Could you check a few things on this model? Use its own coordinates, in mm. Face numbers are marked on the shaded views. Give positions to 0.01 mm unless a question says otherwise; leave off trailing zeros. Order: outer loops, then holes, each group sorted by start corner. A loop starts at its lowest first (then second) coordinate and runs counter-clockwise, first axis right, second up. Notation, with made-up numbers: (33, -10.75) -> (50, -10.75) arc R29 ccw to (50, 17.25) -> close; hole circle Ø4 at (55.25, -13). An arc over 180 degrees is marked (long way). Answer as CSV lines item,"result". Start each with the question number.
(1) Will these pins go through, and if not, where does the flat tip stop? pin 1 Ø1.5 at (x, y) = (18.5, -11) entering from -Z; pin 2 Ø6 at (x, z) = (25.5, 29) entering from +Y; pin 3 Ø6 at (y, z) = (-12, 1.5) entering from +X; pin 4 Ø2.5 at (y, z) = (1.5, 22) entering from -X.
(2) I want a section at A-A (x = 0). Please give me the cut outline in (y, z), plus the area to 3 significant figures.
(3) I want a section at B-B (y = -7). Please give me the cut outline in (x, z).
(4) I need wall thicknesses on L1, parallel to Z at x = 0, y = -10; L2, parallel to Y at x = 14.5, z = -1; L3, parallel to X at y = -4.25, z = 0.5. Which ranges of each line are inside material? Lowest first, please.
(5) We'd pull the mould along X, two halves only. Please class the marked faces 1 and 2: released by +X, released by -X, zero draft, split by the parting line, or undercut.
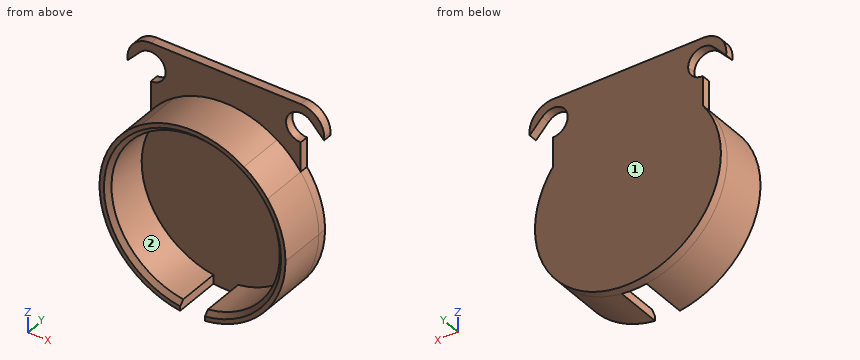
```python
from build123d import *

# Parameters (mm, degrees)
F6_R     = 28.65
F1_DEPTH = 3
F2_DEPTH = 16
F4_DEPTH = 16
F5_SIZE  = 1.5


with BuildPart() as f1:
    # F6 (on Front) → F1 (new body)
    with BuildSketch(Plane.XZ):
        with BuildLine():
            ThreePointArc((-25.5, 18.7475998464), (-9.8652800264, -30.0732231395), (31.65, 0))
            ThreePointArc((31.65, 0), (30.0732231395, 9.8652800264), (25.5, 18.7475998464))
            ThreePointArc((25.5, 18.7475998464), (21.8353418806, 22.9115766581), (17.5, 26.3718126036))
            ThreePointArc((17.5, 26.3718126036), (0, 31.65), (-17.5, 26.3718126036))
            ThreePointArc((-17.5, 26.3718126036), (-21.8353418806, 22.9115766581), (-25.5, 18.7475998464))
        make_face()
        Circle(F6_R, mode=Mode.SUBTRACT)
        Circle(F6_R)
        with BuildLine():
            ThreePointArc((-17.5, 26.3718126036), (0, 31.65), (17.5, 26.3718126036))
            Line((17.5, 26.3718126036), (17.5, 33.7475998464))
            ThreePointArc((17.5, 33.7475998464), (19.8431457505, 39.4044540959), (25.5, 41.7475998464))
            Line((25.5, 41.7475998464), (-25.5, 41.7475998464))
            ThreePointArc((-25.5, 41.7475998464), (-19.8431457505, 39.4044540959), (-17.5, 33.7475998464))
            Line((-17.5, 33.7475998464), (-17.5, 26.3718126036))
        make_face()
        with BuildLine():
            Line((-25.5, 28.7475998464), (-25.5, 25.7475998464))
            ThreePointArc((-25.5, 25.7475998464), (-19.8431457505, 28.0907455969), (-17.5, 33.7475998464))
            ThreePointArc((-17.5, 33.7475998464), (-19.8431457505, 39.4044540959), (-25.5, 41.7475998464))
            ThreePointArc((-25.5, 41.7475998464), (-31.5363482338, 38.9975998464), (-33.4227070569, 32.6382248464))
            Line((-33.4227070569, 32.6382248464), (-29.1360609327, 37.1796634958))
            ThreePointArc((-29.1360609327, 37.1796634958), (-23.6534227154, 38.3941203006), (-20.5, 33.7475998464))
            ThreePointArc((-20.5, 33.7475998464), (-21.9644660941, 30.2120659404), (-25.5, 28.7475998464))
        make_face()
        with BuildLine():
            ThreePointArc((17.5, 33.7475998464), (19.8431457505, 28.0907455969), (25.5, 25.7475998464))
            Line((25.5, 25.7475998464), (25.5, 28.7475998464))
            ThreePointArc((25.5, 28.7475998464), (20.9086865579, 35.7274586485), (29.1360609327, 37.1796634958))
            Line((29.1360609327, 37.1796634958), (33.4227070569, 32.6382248464))
            ThreePointArc((33.4227070569, 32.6382248464), (33.480653371, 33.1915676779), (33.5, 33.7475998464))
            ThreePointArc((33.5, 33.7475998464), (31.1568542495, 39.4044540959), (25.5, 41.7475998464))
            ThreePointArc((25.5, 41.7475998464), (19.8431457505, 39.4044540959), (17.5, 33.7475998464))
        make_face()
        with BuildLine():
            Line((-25.5, 25.7475998464), (-25.5, 18.7475998464))
            ThreePointArc((-25.5, 18.7475998464), (-21.8353418806, 22.9115766581), (-17.5, 26.3718126036))
            Line((-17.5, 26.3718126036), (-17.5, 33.7475998464))
            ThreePointArc((-17.5, 33.7475998464), (-19.8431457505, 28.0907455969), (-25.5, 25.7475998464))
        make_face()
        with BuildLine():
            ThreePointArc((17.5, 26.3718126036), (21.8353418806, 22.9115766581), (25.5, 18.7475998464))
            Line((25.5, 18.7475998464), (25.5, 25.7475998464))
            ThreePointArc((25.5, 25.7475998464), (19.8431457505, 28.0907455969), (17.5, 33.7475998464))
            Line((17.5, 33.7475998464), (17.5, 26.3718126036))
        make_face()
    extrude(amount=-F1_DEPTH)

    # F6 (on Front) → F2 (join)
    with BuildSketch(Plane.XZ):
        with BuildLine():
            ThreePointArc((-25.5, 18.7475998464), (-9.8652800264, -30.0732231395), (31.65, 0))
            ThreePointArc((31.65, 0), (30.0732231395, 9.8652800264), (25.5, 18.7475998464))
            ThreePointArc((25.5, 18.7475998464), (21.8353418806, 22.9115766581), (17.5, 26.3718126036))
            ThreePointArc((17.5, 26.3718126036), (0, 31.65), (-17.5, 26.3718126036))
            ThreePointArc((-17.5, 26.3718126036), (-21.8353418806, 22.9115766581), (-25.5, 18.7475998464))
        make_face()
        Circle(F6_R, mode=Mode.SUBTRACT)
    extrude(amount=F2_DEPTH)

    # F3 (on face) → F4 (cut, through all)
    with BuildSketch(Plane.XZ.offset(16)):
        with BuildLine():
            ThreePointArc((4.2, -28.3404745902), (0, -28.65), (-4.2, -28.3404745902))
            Line((-4.2, -28.3404745902), (-4.2, -31.3700892571))
            ThreePointArc((-4.2, -31.3700892571), (0, -31.65), (4.2, -31.3700892571))
            Line((4.2, -31.3700892571), (4.2, -28.3404745902))
        make_face()
    extrude(amount=-F4_DEPTH, mode=Mode.SUBTRACT)

    # F5
    f5_edges = [f1.edges().sort_by_distance(p)[0] for p in [
        (-18.714867, -16, 21.69277),
    ]]
    chamfer(f5_edges, length=F5_SIZE)


solid = f1.part
```
Final values:
1,pin 1,"z = -26.2"
1,pin 2,"y = 3"
1,pin 3,"x = 31.65"
1,pin 4,"x = -25.5"
2,outline,"(-16, 30.15) -> (-14.5, 28.65) -> (0, 28.65) -> (0, -31.65) -> (3, -31.65) -> (3, 41.75) -> (0, 41.75) -> (0, 31.65) -> (-16, 31.65) -> close"
2,area,"267 mm²"
3,outline,"(-4.2, -31.37) -> (-4.2, -28.34) arc R28.65 cw (long way) to (4.2, -28.34) -> (4.2, -31.37) arc R31.65 ccw (long way) to start"
4,L1,"28.65 to 31.65"
4,L2,"0 to 3"
4,L3,"-31.65 to -28.65, 28.65 to 31.65"
5,face 1,"zero draft"
5,face 2,"undercut"
